The figure shows three views and two pictorial views of one solid part (mm, origin at its lowest corner). Answer the questions. A direction names the side the tool comes from. Coordinates: 2 decimals unless noted, no trailing zeros. Order: outer loops, then holes, each group sorted by start corner. A loop starts at its lowest first (then second) coordinate and runs counter-clockwise, first axis right, second up. Notation, with made-up numbers: (40, 34.5) - (72, 34.5) arc R14 ccw to (72, 48.5) - close; hole circle Ø5 at (57.5, 61.5). An arc over 180 degrees is marked (long way). Use one line per item in the form item = value.
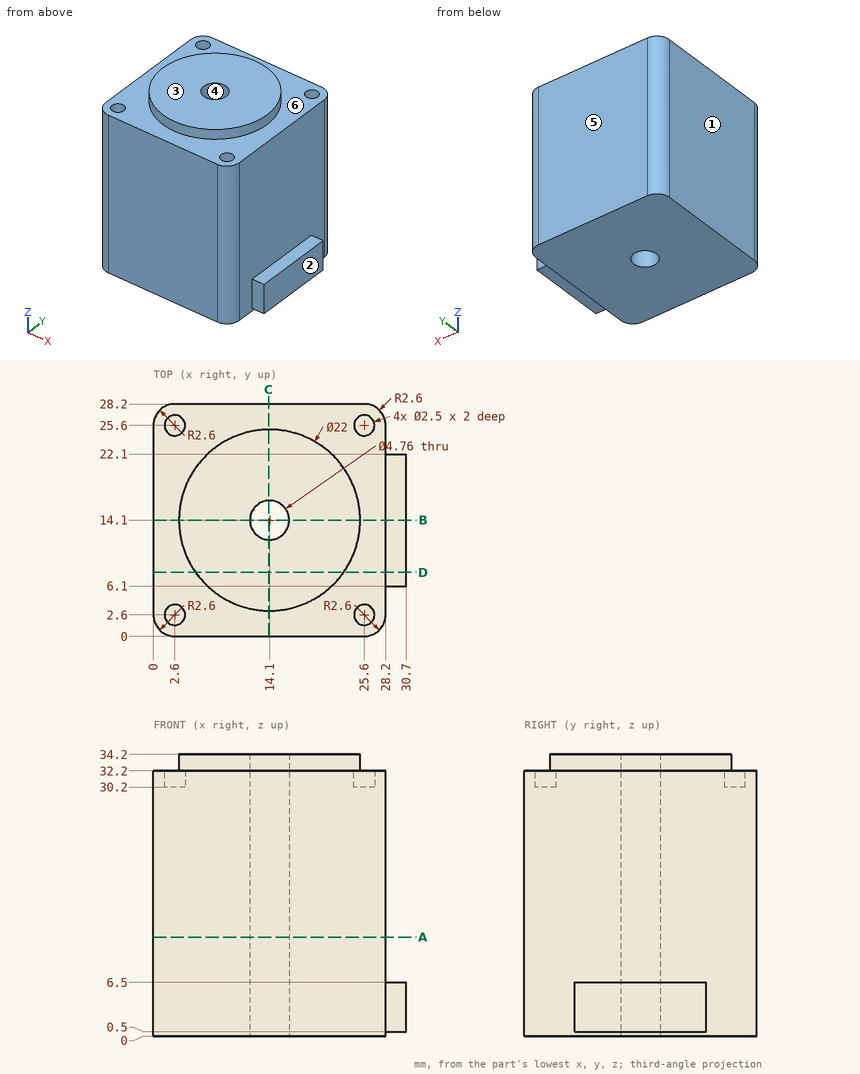
(1) Given pin 1 Ø3 at (x, y) = (30, 13) entering from -Z; pin 2 Ø1.2 at (x, y) = (29, 16) entering from +Z; pin 3 Ø1.3 at (x, z) = (29.5, 5) entering from -Y; pin 4 Ø3 at (x, y) = (14.1, 14.1) entering from +Z, each flat-ended and moving along its own axis, determine where each tip first touches the part or whether it passes through.
Answer list:
pin_1 = 0.5
pin_2 = 6.5
pin_3 = 6.1
pin_4 = through
(2) Which of the six approach directions +Z, -Z, +X, -X, +Y, -Y give full straight-line access (tool end or side, diameter ignored) to the marked faces 5 and 6?
Answer list:
face_5 = +Z, -Z, +X, -X, +Y
face_6 = +Z
(3) Section D-D, the plane y = 7.75 is taken. Write down the section's boundary in (x, z).
Answer list:
outline = (0, 0) - (28.2, 0) - (28.2, 0.5) - (30.7, 0.5) - (30.7, 6.5) - (28.2, 6.5) - (28.2, 32.2) - (23.08, 32.2) - (23.08, 34.2) - (5.12, 34.2) - (5.12, 32.2) - (0, 32.2) - close
(4) Section B-B, the plane y = 14.1 is taken. Write down the section's boundary in (x, z).
Answer list:
outline = (0, 0) - (11.72, 0) - (11.72, 34.2) - (3.1, 34.2) - (3.1, 32.2) - (0, 32.2) - close; (16.48, 0) - (28.2, 0) - (28.2, 0.5) - (30.7, 0.5) - (30.7, 6.5) - (28.2, 6.5) - (28.2, 32.2) - (25.1, 32.2) - (25.1, 34.2) - (16.48, 34.2) - close
(5) Section C-C, the plane x = 14 is taken. Write down the section's boundary in (y, z).
Answer list:
outline = (0, 0) - (11.72, 0) - (11.72, 34.2) - (3.1, 34.2) - (3.1, 32.2) - (0, 32.2) - close; (16.48, 0) - (28.2, 0) - (28.2, 32.2) - (25.1, 32.2) - (25.1, 34.2) - (16.48, 34.2) - close
(6) Section A-A, the plane z = 12 is taken. Write down the section's boundary in (x, y), then the cut area to 3 significant figures.
Answer list:
outline = (0, 2.6) arc R2.6 ccw to (2.6, 0) - (25.6, 0) arc R2.6 ccw to (28.2, 2.6) - (28.2, 25.6) arc R2.6 ccw to (25.6, 28.2) - (2.6, 28.2) arc R2.6 ccw to (0, 25.6) - close; hole circle Ø4.76 at (14.1, 14.1)
area = 772 mm2
(7) Straight lines are drawn through the part: L1, parallel to Y at x = 25.6, z = 31.2; L2, parallel to Z at x = 4, y = 5.25; L3, parallel to Y at x = 2, z = 31. For each, find the intervals that lie inside material, in ascending order.
Answer list:
L1 = 0 to 1.35, 3.85 to 24.35, 26.85 to 28.2
L2 = 0 to 32.2
L3 = 0.07 to 1.5, 3.7 to 24.5, 26.7 to 28.13
(8) The mould has two halves that part along X. Classify the marked faces 1, 2, 3 and 4: +X half, -X half, draft (parallel to the pull), parting line (faces both ways), or undercut.
Answer list:
face_1 = -X half
face_2 = +X half
face_3 = draft
face_4 = undercut
